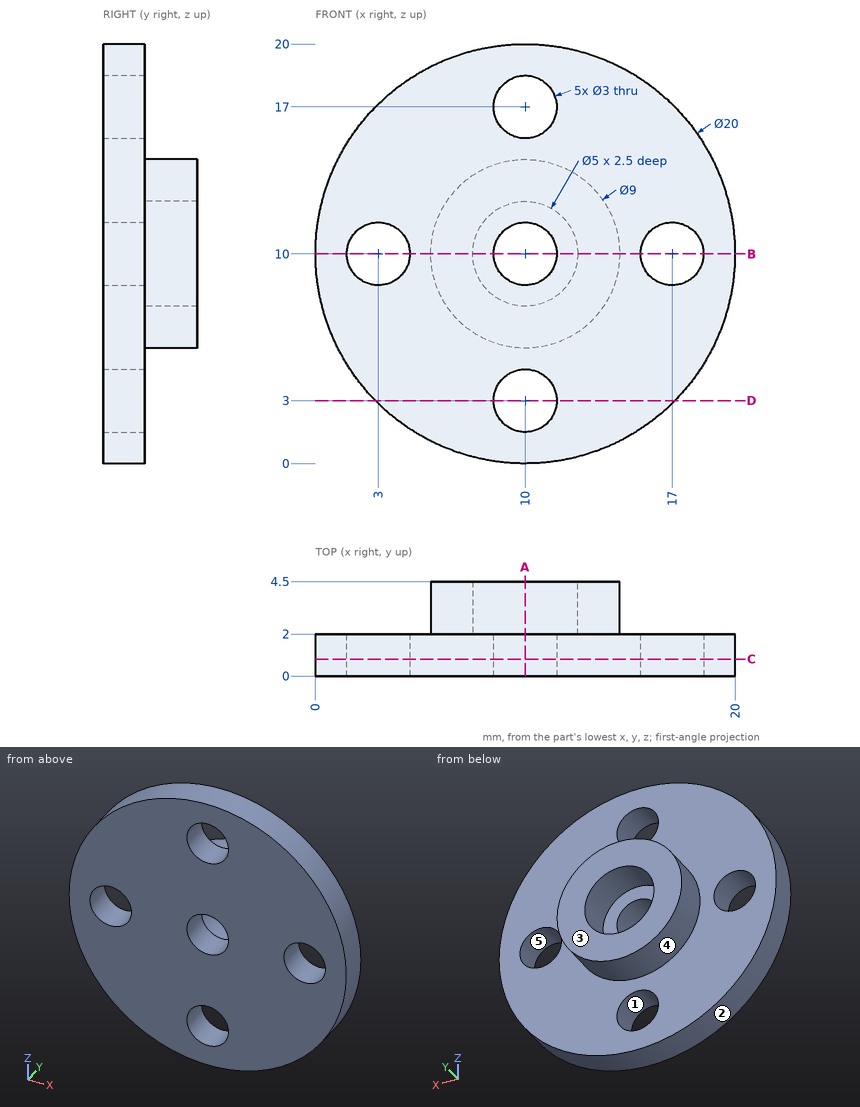
The drawing under review shows one solid part. Ordinate dimensions are in mm from its lowest x, y, z. A direction names the side the tool comes from. Round coordinates to 2 decimals unless told otherwise and drop trailing zeros. Order: outer loops, then holes, each group sorted by start corner. A loop starts at its lowest first (then second) coordinate and runs counter-clockwise, first axis right, second up. Notation, with made-up numbers: (28.25, 68) - (85.25, 68) arc R25 cw to (85.25, 107) - close; hole circle Ø2 at (27.5, 46.5). An arc over 180 degrees is marked (long way). Return JSON: item names as keys, results as strings.
Q1. Consider section B-B on z = 10. Write out the cut boundary in (x, y).
Computed values:
{"outline": "(0, 0) - (1.5, 0) - (1.5, 2) - (0, 2) - close; (4.5, 0) - (8.5, 0) - (8.5, 2) - (7.5, 2) - (7.5, 4.5) - (5.5, 4.5) - (5.5, 2) - (4.5, 2) - close; (11.5, 0) - (15.5, 0) - (15.5, 2) - (14.5, 2) - (14.5, 4.5) - (12.5, 4.5) - (12.5, 2) - (11.5, 2) - close; (18.5, 0) - (20, 0) - (20, 2) - (18.5, 2) - close"}
Q2. Consider section C-C on y = 0.8. Write out the cut boundary in (x, z).
Computed values:
{"outline": "circle Ø20 at (10, 10); hole circle Ø3 at (3, 10); hole circle Ø3 at (10, 3); hole circle Ø3 at (10, 10); hole circle Ø3 at (10, 17); hole circle Ø3 at (17, 10)"}
Q3. The part is to be moulded in two halves that separate along X. For the marked faces 1, 2 and 3, say which applies: pulls with the +X half, pulls with the -X half, needs draft (parallel to the pull), parting line crosses it, or undercut.
Computed values:
{"face 1": "undercut", "face 2": "parting line crosses it", "face 3": "needs draft"}
Q4. Consider section A-A on x = 10. Write out the cut boundary in (y, z), plus the area to 3 significant figures.
Computed values:
{"outline": "(0, 0) - (2, 0) - (2, 1.5) - (0, 1.5) - close; (0, 4.5) - (2, 4.5) - (2, 5.5) - (4.5, 5.5) - (4.5, 7.5) - (2, 7.5) - (2, 8.5) - (0, 8.5) - close; (0, 11.5) - (2, 11.5) - (2, 12.5) - (4.5, 12.5) - (4.5, 14.5) - (2, 14.5) - (2, 15.5) - (0, 15.5) - close; (0, 18.5) - (2, 18.5) - (2, 20) - (0, 20) - close", "area": "32.0 mm2"}
Q5. Consider section D-D on z = 3. Write out the cut boundary in (x, y).
Computed values:
{"outline": "(2.86, 0) - (8.5, 0) - (8.5, 2) - (2.86, 2) - close; (11.5, 0) - (17.14, 0) - (17.14, 2) - (11.5, 2) - close"}
Q6. For pin 1 Ø1.5 at (y, z) = (2.5, 12) entering from +X; pin 2 Ø1 at (x, y) = (4, 1.5) entering from +Z; pin 3 Ø1.5 at (y, z) = (2.5, 11) entering from +X, all flat-tipped, find the tip position at first contact; note any pin that passes through.
Computed values:
{"pin 1": "stops at x = 19.9", "pin 2": "stops at z = 18.35", "pin 3": "stops at x = 19.99"}
Q7. Machinability: for the marked faces 4 and 5, which of the approach directions +Z, -Z, +X, -X, +Y, -Y give a long, thin tool a straight path to every point of the face, cutting with its end or side? Answer none if there is none.
Computed values:
{"face 4": "+Y", "face 5": "+Y, -Y"}
Q8. Wall thickness on L1, parallel to X at y = 0.8, z = 10; L2, parallel to Z at x = 10, y = 2.95: over which ranges is each line inside the solid? List them lowest first. Write a range as [from, to].
Computed values:
{"L1": "x = [0, 1.5], [4.5, 8.5], [11.5, 15.5], [18.5, 20]", "L2": "z = [5.5, 7.5], [12.5, 14.5]"}
